The listing builds one solid part. Answer for the finished solid, in the listing's coordinates (mm). Face numbers are marked on the shaded views. A direction names the side the tool comes from. Give positions to 0.01 mm unless a question says otherwise; leave off trailing zeros. Write each loop counter-clockwise with the first axis right and the second up, starting at its lowest first coordinate (ties: lowest second). Pieces come first, ordered by that corner, then holes.
```python
from build123d import *

# Parameters (mm, degrees)
SKETCH1_W           = 55
SKETCH1_H           = 55
BOSS_EXTRUDE1_DEPTH = 5
LOFT1_START         = -7.5
LOFT1_DEPTH         = 15
SKETCH7_R           = 3.15
CUT_EXTRUDE1_DEPTH  = 42.683330037
BOSS_EXTRUDE2_DEPTH = 15
SKETCH10_R          = 2
CUT_EXTRUDE2_DEPTH  = 69.855497331


# Read off the part's stored shape, not the designer's step: Loft1
with BuildPart() as part:
    # Sketch1 → Boss-Extrude1 (new body)
    with BuildSketch(Plane(origin=(0, 0, 0), x_dir=(1, 0, 0), z_dir=(0, 1, 0))):
        Rectangle(SKETCH1_W, SKETCH1_H)
    extrude(amount=BOSS_EXTRUDE1_DEPTH)

    # Loft1 outline → Loft1 (add)
    with BuildSketch(Plane.XY.offset(LOFT1_START)):
        with BuildLine():
            add(Edge.make_bspline(
                [(2.5, 15), (2.5, 10.833333333), (6.25, 7.916666667), (10, 5)],
                knots=[0, 0, 0, 0, 1, 1, 1, 1], degree=3))
            Line((2.5, 15), (-2.5, 15))
            add(Edge.make_bspline(
                [(-2.5, 15), (-2.5, 10.833333333), (-6.25, 7.916666667), (-10, 5)],
                knots=[0, 0, 0, 0, 1, 1, 1, 1], degree=3))
            Line((-10, 5), (10, 5))
        make_face()
    extrude(amount=LOFT1_DEPTH)

    # Sketch7 → Cut-Extrude1 (cut, through all)
    with BuildSketch(Plane(origin=(0, 0, 0), x_dir=(-1, 0, 0), z_dir=(0, -1, 0))):
        with Locations(Location((23.5, -23.5, 0), (0, 0, 90))):
            Circle(SKETCH7_R)
        with Locations(Location((-23.5, -23.5, 0), (0, 0, 90))):
            Circle(SKETCH7_R)
        with Locations(Location((-23.5, 23.5, 0), (0, 0, 90))):
            Circle(SKETCH7_R)
        with Locations(Location((23.5, 23.5, 0), (0, 0, 90))):
            Circle(SKETCH7_R)
    extrude(amount=-CUT_EXTRUDE1_DEPTH, mode=Mode.SUBTRACT)

    # Sketch8 → Boss-Extrude2 (add)
    with BuildSketch(Plane(origin=(0, 0, -7.5), x_dir=(-1, 0, 0), z_dir=(0, 0, -1))):
        with BuildLine():
            Line((-10.386332084, 31.349499896), (-10.386332084, 46.349499896))
            Line((-10.386332084, 46.349499896), (-15.355027277, 46.349499896))
            Line((-15.355027277, 46.349499896), (-15.355027277, 31.349499896))
            ThreePointArc((-15.355027277, 31.349499896), (0, 11.24185629), (15.355027277, 31.349499896))
            Line((15.355027277, 31.349499896), (15.355027277, 46.349499896))
            Line((15.355027277, 46.349499896), (10.386332084, 46.349499896))
            Line((10.386332084, 46.349499896), (10.386332084, 31.349499896))
            ThreePointArc((10.386332084, 31.349499896), (10.968139681, 29.425682042), (11.196737575, 27.428855004))
            ThreePointArc((11.196737575, 27.428855004), (11.085843409, 25.563528692), (10.666364419, 23.742601142))
            ThreePointArc((10.666364419, 23.742601142), (0, 15.958544655), (-10.666364419, 23.742601142))
            ThreePointArc((-10.666364419, 23.742601142), (-11.048273693, 25.321250886), (-11.197838961, 26.93853872))
            ThreePointArc((-11.197838961, 26.93853872), (-11.015137518, 29.185055314), (-10.386332084, 31.349499896))
        make_face()
    extrude(amount=-BOSS_EXTRUDE2_DEPTH)

    # Sketch10 → Cut-Extrude2 (cut, through all)
    with BuildSketch(Plane(origin=(15.355027277, 0, 0), x_dir=(0, 0, -1), z_dir=(1, 0, 0))):
        with Locations(Location((0, 42.349499896, 0), (0, 0, 180))):
            Circle(SKETCH10_R)
    extrude(amount=-CUT_EXTRUDE2_DEPTH, mode=Mode.SUBTRACT)


solid = part.part
```
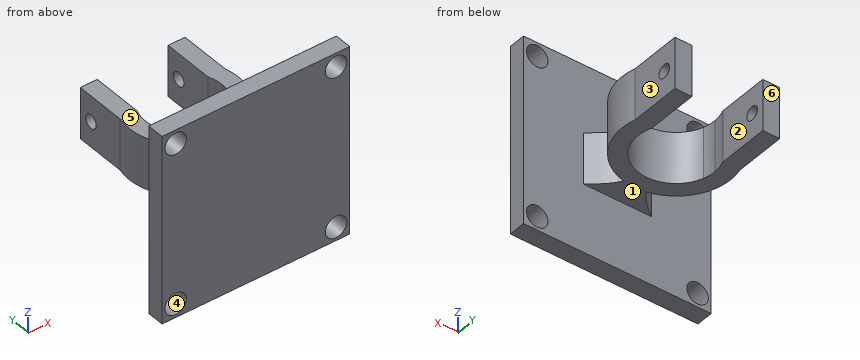
Item 1: A cutting plane is placed at D-D, the plane x = 14.5. Give the vertices of the cut face in (y, z).
Conclusion:
outline: (0, -27.5) - (5, -27.5) - (5, 27.5) - (0, 27.5) - close; (20.59, -7.5) - (46.35, -7.5) - (46.35, 7.5) - (20.59, 7.5) - close; hole circle Ø4 at (42.35, 0)
Item 2: Each of these flat-tipped pins is pushed along its axis until it touches: P1, Ø4, axis at y = 8, z = 11, coming from the -X side; P2, Ø16.5, axis at y = 35.5, z = 2.5, coming from the +X side; P3, Ø10, axis at x = -23.5, z = 23.5, coming from the +Y side; P4, Ø16.5, axis at y = 41.5, z = -2.5, coming from the -X side (3 decimals). Where does it stop, or does it pass through?
Conclusion:
P1: passes through
P2: stops at x = 15.92
P3: stops at y = 5
P4: stops at x = -15.355
Item 3: A cutting plane is placed at C-C, the plane y = 37. Give the vertices of the cut face in (x, z).
Conclusion:
outline: (-15.36, -7.5) - (-10.39, -7.5) - (-10.39, 7.5) - (-15.36, 7.5) - close; (10.39, -7.5) - (15.36, -7.5) - (15.36, 7.5) - (10.39, 7.5) - close
Item 4: A cutting plane is placed at A-A, the plane x = 23.5. Give the vertices of the cut face in (y, z).
Conclusion:
outline: (0, -27.5) - (5, -27.5) - (5, -26.65) - (0, -26.65) - close; (0, -20.35) - (5, -20.35) - (5, 20.35) - (0, 20.35) - close; (0, 26.65) - (5, 26.65) - (5, 27.5) - (0, 27.5) - close
Item 5: A cutting plane is placed at B-B, the plane z = 23.5. Give the vertices of the cut face in (x, y), plus the area to 3 significant figures.
Conclusion:
outline: (-27.5, 0) - (-26.65, 0) - (-26.65, 5) - (-27.5, 5) - close; (-20.35, 0) - (20.35, 0) - (20.35, 5) - (-20.35, 5) - close; (26.65, 0) - (27.5, 0) - (27.5, 5) - (26.65, 5) - close
area: 212 mm2
Item 6: Determine the mould class of the marked faces 4, 5 and 6 for opening direction Z: pulls with the +Z half, pulls with the -Z half, needs draft (parallel to the pull), parting line crosses it, or undercut.
Conclusion:
face 4: undercut
face 5: pulls with the +Z half
face 6: needs draft
Item 7: Consider probe 1 along X at (y, z) = (3.35, -23.5); probe 2 along Y at (x, z) = (0.5, 18); probe 3 along X at (y, z) = (44.5, -5). Determine where each line is inside the solid, lowest interval first.
Conclusion:
probe 1: x = -27.5 to -26.65, -20.35 to 20.35, 26.65 to 27.5
probe 2: y = 0 to 5
probe 3: x = -15.36 to -10.39, 10.39 to 15.36
Item 8: Which of the six approach directions +Z, -Z, +X, -X, +Y, -Y give full straight-line access (tool end or side, diameter ignored) to the marked faces 1, 2 and 3?
Conclusion:
face 1: -Z, +X, -X, +Y
face 2: +Z, -Z, +Y
face 3: +Z, -Z, +X, +Y
